Could you check a few things on this model? Use its own coordinates, in mm. Face numbers are marked on the shaded views. A direction names the side the tool comes from. Round coordinates to 2 decimals unless told otherwise and drop trailing zeros. Loops run counter-clockwise (first coordinate to the right, second up) from the corner with the lowest first, then second, coordinate; pieces in that order, holes last. Notation, with made-up numbers: (49.25, -12.75) -> (76.25, -12.75) arc R22 cw to (76.25, -5.75) -> close; hole circle Ø11 at (-19, -39). An arc over 180 degrees is marked (long way). One line per item, written item: value.
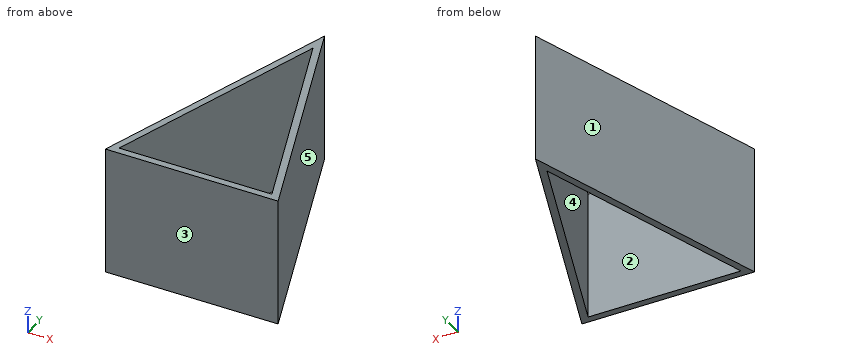
```python
from build123d import *

# Parameters (mm, degrees)
F1_DEPTH = 36.83


with BuildPart() as f1:
    # F0 (on Top) → F1 (new body)
    with BuildSketch(Plane.XY):
        Polygon((26.076875, -28.768841), (-0.115304, 43.006679), (-23.342333, -28.768841), align=None)
        Polygon((-20.549016, -26.736841), (0, 36.763159), (23.172293, -26.736841), (0, -26.736841), align=None, mode=Mode.SUBTRACT)
    extrude(amount=F1_DEPTH)


solid = f1.part
```
Item 1: If we section it at D-D on y = 38.5: List the corners of the cut face in (x, z) for me, plus the area to 3 significant figures.
Output:
outline: (-1.57, 0) -> (1.53, 0) -> (1.53, 36.83) -> (-1.57, 36.83) -> close
area: 114 mm²
Item 2: I need wall thicknesses on line 1 (X direction, y = 35, z = 32); line 2 (X direction, y = -4, z = 19); line 3 (X direction, y = 40.5, z = 32). Which ranges of each line are inside material? Lowest first, please. Write a range as from..to.
Output:
line 1: x = -2.71..-0.57, 0.64..2.81
line 2: x = -15.33..-13.19, 14.88..17.04
line 3: x = -0.93..0.8
Item 3: If we section it at A-A on y = -19: List the corners of the cut face in (x, z) for me, plus the area to 3 significant figures.
Output:
outline: (-20.18, 0) -> (-18.05, 0) -> (-18.05, 36.83) -> (-20.18, 36.83) -> close; (20.35, 0) -> (22.51, 0) -> (22.51, 36.83) -> (20.35, 36.83) -> close
area: 158 mm²
Item 4: For the marked faces 1 and 2, which set-ups out of +Z, -Z, +X, -X, +Y, -Y let a thin tool reach every point of the face, with its end or its side?
Output:
face 1: +Z, -Z, -X, +Y
face 2: +Z, -Z
Item 5: If we section it at C-C on z = 25: List the corners of the cut face in (x, y) for me, plus the area to 3 significant figures.
Output:
outline: (-23.34, -28.77) -> (26.08, -28.77) -> (-0.12, 43.01) -> close; hole (-20.55, -26.74) -> (23.17, -26.74) -> (0, 36.76) -> close
area: 385 mm²
Item 6: If we mould it in two halves opening along Y, with no side actions, what happens to the marked faces 3, 4 and 5? For each: released by +Y, released by -Y, zero draft, split by the parting line, or undercut.
Output:
face 3: released by -Y
face 4: undercut
face 5: released by +Y
Item 7: Will these pins go through, and if not, where does the flat tip stop? pin 1 Ø4 at (x, y) = (-14.5, 4.5) entering from +Z; pin 2 Ø12 at (y, z) = (28, 9) entering from +X.
Output:
pin 1: stops at z = 36.83
pin 2: stops at x = 7.55
Item 8: If we section it at B-B on x = -11.5: List the corners of the cut face in (y, z) for me.
Output:
outline: (-28.77, 0) -> (-26.74, 0) -> (-26.74, 36.83) -> (-28.77, 36.83) -> close; (1.23, 0) -> (7.83, 0) -> (7.83, 36.83) -> (1.23, 36.83) -> close
